The figure shows three views and two pictorial views of one solid part (mm, origin at its lowest corner). Answer the questions. Give positions to 0.01 mm unless a question says otherwise; leave off trailing zeros. Loops run counter-clockwise (first coordinate to the right, second up) from the corner with the lowest first, then second, coordinate; pieces in that order, holes last. Notation, with made-up numbers: (71.25, -11.75) - (113.25, -11.75) arc R11 ccw to (113.25, -3.75) - close; hole circle Ø3 at (63, 2). An arc over 180 degrees is marked (long way). Write each question's results on one line, items separated by ' | '.
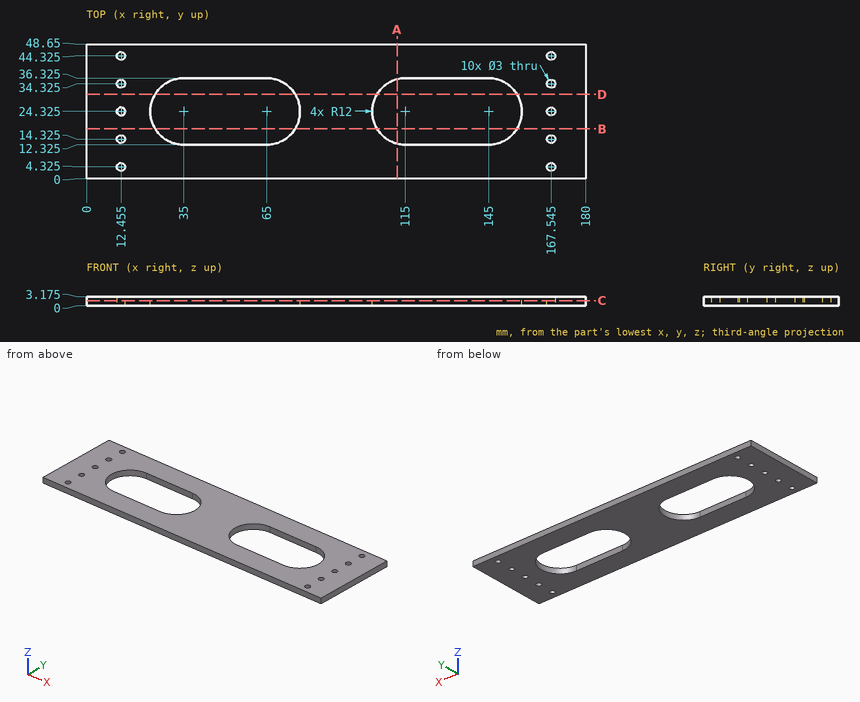
Item 1: A cutting plane is placed at C-C, the plane z = 1.8. Count the separate pieces of the cut face and the enclosed holes in it, plus the area to 3 significant figures.
Values found:
separate pieces: 1 | enclosed holes: 12 | area: 6,340 mm²
Item 2: A cutting plane is placed at A-A, the plane x = 112. Determine the outline of the cut face in (y, z) (3 decimals).
Values found:
outline: (0, 0) - (12.706, 0) - (12.706, 3.175) - (0, 3.175) - close; (35.944, 0) - (48.65, 0) - (48.65, 3.175) - (35.944, 3.175) - close
Item 3: Flat-ended cylindrical pins translate along their axes: P1, Ø2.5, axis at x = 167.545, y = 34.325, coming from the -Z side; P2, Ø1, axis at x = 48.5, z = 1, coming from the -Y side. Find the tip coordinate at first contact, or state that the pin passes through.
Values found:
P1: passes through | P2: stops at y = 0
Item 4: Find the intervals of material crossed by line 1 along X through (y, z) = (44.5, 1.15); line 2 along Y through (x, z) = (140, 0.8) (3 decimals); line 3 along X through (y, z) = (23, 1.3), in increasing order. Write a range as [from, to].
Values found:
line 1: x = [0, 10.97], [13.94, 166.06], [169.03, 180] | line 2: y = [0, 12.325], [36.325, 48.65] | line 3: x = [0, 11.75], [13.16, 23.07], [76.93, 103.07], [156.93, 166.84], [168.25, 180]
Item 5: A cutting plane is placed at D-D, the plane y = 30.5. Determine the outline of the cut face in (x, z) (3 decimals).
Values found:
outline: (0, 0) - (24.711, 0) - (24.711, 3.175) - (0, 3.175) - close; (75.289, 0) - (104.711, 0) - (104.711, 3.175) - (75.289, 3.175) - close; (155.289, 0) - (180, 0) - (180, 3.175) - (155.289, 3.175) - close
Item 6: A cutting plane is placed at B-B, the plane y = 18. Determine the outline of the cut face in (x, z) (3 decimals).
Values found:
outline: (0, 0) - (24.802, 0) - (24.802, 3.175) - (0, 3.175) - close; (75.198, 0) - (104.802, 0) - (104.802, 3.175) - (75.198, 3.175) - close; (155.198, 0) - (180, 0) - (180, 3.175) - (155.198, 3.175) - close
